```python
from build123d import *

# Parameters (mm, degrees)
CORNERBOSS_EXTRUDE1_DEPTH               = 20
SHELL2_T                                = -3
PADSKETCH3_R                            = 12
PADSKETCH3_R_2                          = 5
PADBOSS_EXTRUDE2_DEPTH                  = 10
STEPPERSHAFTHOLESKETCH4_R               = 5.1
STEPPERSHAFTHOLESKETCH4_R_2             = 2
STEPPERSHAFTCUT_EXTRUDE2_DEPTH          = 316.846451025
THREADEDNUTMOUNTHOLESSKETCH5_R          = 2
THREADEDNUTMOUNTHOLESCUT_EXTRUDE4_DEPTH = 10
TRPEGSKETCH1_W                          = 9.8
TRPEGSKETCH1_H                          = 13.9
TRPEGBOSS_EXTRUDE1_DEPTH                = 3.1
TRPEGCAPSKETCH2_W                       = 16
TRPEGCAPSKETCH2_H                       = 17
TRPEGCAPBOSS_EXTRUDE2_DEPTH             = 3
BOTTOMPEGHOLESKETCH3_W                  = 10
BOTTOMPEGHOLESKETCH3_H                  = 13.9
BOTTOMPEGHOLECUT_EXTRUDE1_DEPTH         = 3
BEDCENTERPEGHOLECUTSKETCH1_W            = 10
BEDCENTERPEGHOLECUTSKETCH1_H            = 14
BEDCENTERPEGHOLECUT_EXTRUDE1_DEPTH      = 3


with BuildPart() as part:
    # CornerrSketch1 → CornerBoss-Extrude1 (new body)
    with BuildSketch(Plane(origin=(0, 0, 0), x_dir=(1, 0, 0), z_dir=(0, 1, 0))):
        with BuildLine():
            Line((140, 220), (140, 140))
            Line((140, 140), (70, 140))
            Line((70, 140), (70, 0))
            Line((70, 0), (0, 0))
            Line((0, 0), (0, 265.825))
            ThreePointArc((0, 265.825), (17, 282.825), (34, 265.825))
            Line((34, 265.825), (34, 220))
            Line((34, 220), (140, 220))
        make_face()
    extrude(amount=CORNERBOSS_EXTRUDE1_DEPTH)

    # Shell2
    shell2_openings = [part.faces().sort_by_distance(p)[0] for p in [
        (50.460788317, 0, -139.249856422),
    ]]
    offset(amount=SHELL2_T, openings=shell2_openings, kind=Kind.INTERSECTION)

    # PadSketch3 → PadBoss-Extrude2 (add)
    with BuildSketch(Plane.XZ.offset(-17)):
        with Locations(Location((17, -265.825, 0), (0, 0, 90))):
            Circle(PADSKETCH3_R)
        with Locations((7, -34)):
            Circle(PADSKETCH3_R_2)
    extrude(amount=PADBOSS_EXTRUDE2_DEPTH)

    # StepperShaftHoleSketch4 → StepperShaftCut-Extrude2 (cut, through all)
    with BuildSketch(Plane.XZ.offset(-7)):
        with Locations(Location((17, -265.825, 0), (0, 0, 270))):
            Circle(STEPPERSHAFTHOLESKETCH4_R)
        with Locations(Location((7, -34, 0), (0, 0, 270))):
            Circle(STEPPERSHAFTHOLESKETCH4_R_2)
    extrude(amount=-STEPPERSHAFTCUT_EXTRUDE2_DEPTH, mode=Mode.SUBTRACT)

    # ThreadedNutMountHolesSketch5 → ThreadedNutMountHolesCut-Extrude4 (cut)
    with BuildSketch(Plane(origin=(0, 7, 0), x_dir=(-1, 0, 0), z_dir=(0, -1, 0))):
        with Locations(Location((-17, 273.825, 0), (0, 0, 90))):
            Circle(THREADEDNUTMOUNTHOLESSKETCH5_R)
        with Locations(Location((-9, 265.825, 0), (0, 0, 90))):
            Circle(THREADEDNUTMOUNTHOLESSKETCH5_R)
        with Locations(Location((-17, 257.825, 0), (0, 0, 90))):
            Circle(THREADEDNUTMOUNTHOLESSKETCH5_R)
        with Locations(Location((-25, 265.825, 0), (0, 0, 90))):
            Circle(THREADEDNUTMOUNTHOLESSKETCH5_R)
    extrude(amount=-THREADEDNUTMOUNTHOLESCUT_EXTRUDE4_DEPTH, mode=Mode.SUBTRACT)

    # TRPegSketch1 → TRPegBoss-Extrude1 (add)
    with BuildSketch(Plane(origin=(140, 0, 0), x_dir=(0, 0, -1), z_dir=(1, 0, 0))):
        with Locations((205, 6.95)):
            Rectangle(TRPEGSKETCH1_W, TRPEGSKETCH1_H)
    extrude(amount=TRPEGBOSS_EXTRUDE1_DEPTH)

    # TRPegCapSketch2 → TRPegCapBoss-Extrude2 (add)
    with BuildSketch(Plane(origin=(143.1, 0, 0), x_dir=(0, 0, -1), z_dir=(1, 0, 0))):
        with Locations((205.1, 8.5)):
            Rectangle(TRPEGCAPSKETCH2_W, TRPEGCAPSKETCH2_H)
    extrude(amount=TRPEGCAPBOSS_EXTRUDE2_DEPTH)

    # BottomPegHoleSketch3 → BottomPegHoleCut-Extrude1 (cut)
    with BuildSketch(Plane.XY):
        with Locations((15, 6.95)):
            Rectangle(BOTTOMPEGHOLESKETCH3_W, BOTTOMPEGHOLESKETCH3_H)
    extrude(amount=-BOTTOMPEGHOLECUT_EXTRUDE1_DEPTH, mode=Mode.SUBTRACT)

    # BedCenterPegHoleCutSketch1 → BedCenterPegHoleCut-Extrude1 (cut)
    with BuildSketch(Plane(origin=(70, 0, 0), x_dir=(0, 0, -1), z_dir=(1, 0, 0))):
        with Locations((35, 7)):
            Rectangle(BEDCENTERPEGHOLECUTSKETCH1_W, BEDCENTERPEGHOLECUTSKETCH1_H)
    extrude(amount=-BEDCENTERPEGHOLECUT_EXTRUDE1_DEPTH, mode=Mode.SUBTRACT)


solid = part.part
```
For this review, take the finished solid that the model builds, in its own axes (mm). A direction names the side the tool comes from. Round coordinates to 2 decimals unless told otherwise and drop trailing zeros. Write each loop counter-clockwise with the first axis right and the second up, starting at its lowest first coordinate (ties: lowest second). Pieces come first, ordered by that corner, then holes.
1) Insertion check: pin 1 Ø12 at (x, y) = (119, 10) entering from +Z; pin 2 Ø6 at (x, z) = (17, -265.825) entering from +Y; pin 3 Ø0.9 at (x, z) = (141, -202.5) entering from +Y; pin 4 Ø3 at (x, z) = (17, -274) entering from -Y. Each pin has a flat end and moves straight along its axis. Give the tip position at first contact, or say it passes through.
Answer below:
pin 1: stops at z = -140
pin 2: passes through
pin 3: stops at y = 13.9
pin 4: stops at y = 17
2) Take a section at B-B on z = -87. Give the boundary of the cut face in (x, y), then the cut area to 3 significant figures.
Answer below:
outline: (0, 0) - (3, 0) - (3, 17) - (67, 17) - (67, 0) - (70, 0) - (70, 20) - (0, 20) - close
area: 312 mm2
3) For line 1 along X through (y, z) = (10, -266); line 2 along Z through (x, y) = (115, 16.25); line 3 along X through (y, z) = (11.5, -160), list the stretches that pass through material, from the lowest coordinate up.
Answer below:
line 1: x = 0 to 3, 5 to 7.01, 10.99 to 11.9, 22.1 to 23.01, 26.99 to 29, 31 to 34
line 2: z = -220 to -217, -143 to -140
line 3: x = 0 to 3, 137 to 140
4) Take a section at A-A on x = 122.5. Give the boundary of the cut face in (y, z).
Answer below:
outline: (0, -220) - (20, -220) - (20, -140) - (0, -140) - (0, -143) - (17, -143) - (17, -217) - (0, -217) - close
5) Machinability: for faces 1 (the face through (35, 10, 0)), 2 (the face through (35, 8, -3)), 3 (the face through (86, 10, -220)), 4 (the face through (143.1, 14.3, -205)), 5 (the face through (55, 20, -143)), which of the approach directions +Z, -Z, +X, -X, +Y, -Y give a long, thin tool a straight path to every point of the face, cutting with its end or side? Answer none if there is none.
Answer below:
face 1: +Z, +X, -X, +Y, -Y
face 2: -Y
face 3: -Z, +X, +Y, -Y
face 4: +Y
face 5: +Z, -Z, +X, -X, +Y
6) Mouldability with a two-part tool opening along X and no side actions: class faces 6 (the face through (67, 8, -74)), 7 (the face through (146.1, 9, -205)), 8 (the face through (0, 10, -131)), 9 (the face through (67.3, 0, -140.8)) as +X half, -X half, draft (parallel to the pull), parting line (faces both ways), or undercut.
Answer below:
face 6: undercut
face 7: +X half
face 8: -X half
face 9: draft
